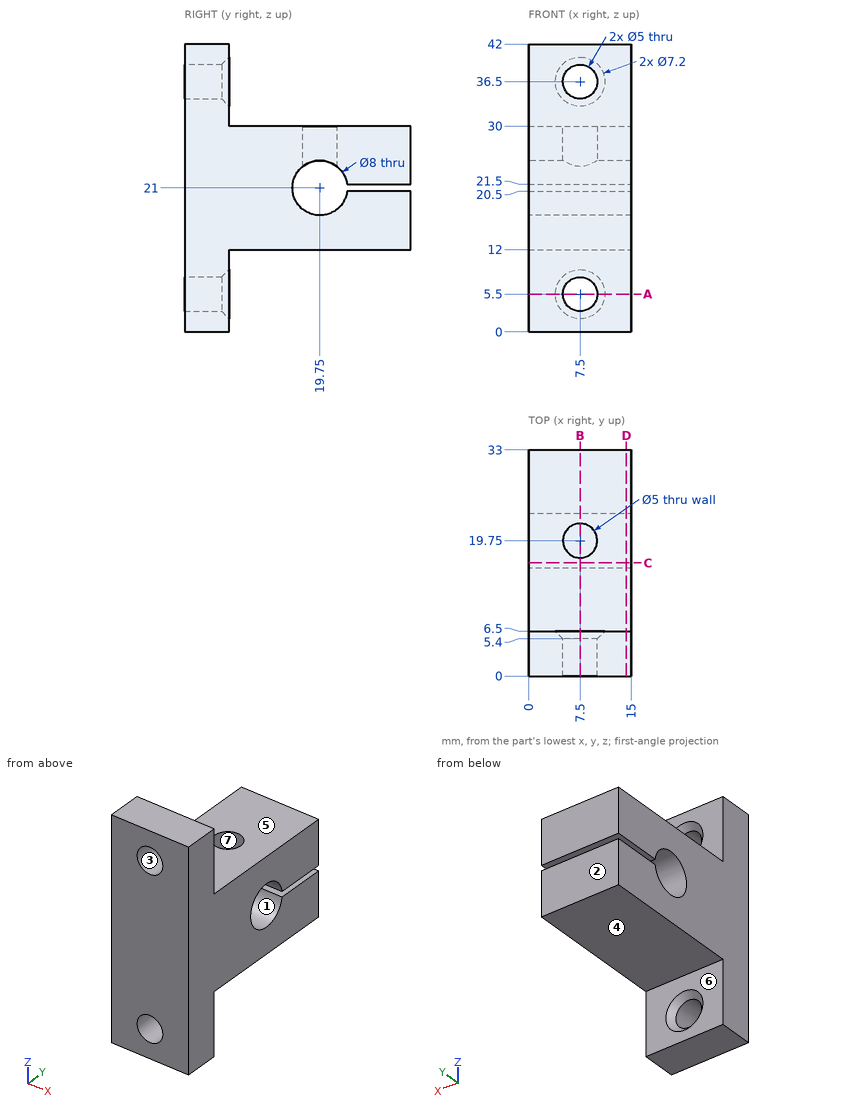
Answer from the drawing. Dimensions are ordinates in mm from the lowest x, y and z of the part. A direction names the side the tool comes from. Round coordinates to 2 decimals unless told otherwise and drop trailing zeros. Loops run counter-clockwise (first coordinate to the right, second up) from the corner with the lowest first, then second, coordinate; pieces in that order, holes last.
(1) Each of these flat-tipped pins is pushed along its axis until it touches: P1, Ø1, axis at x = 11.5, y = 28, coming from the -Z side; P2, Ø1.5, axis at x = 5.5, y = 10.5, coming from the +Z side; P3, Ø3, axis at x = 7.5, y = 19.75, coming from the +Z side. Where does it stop, or does it pass through?
Computed values:
P1: stops at z = 12
P2: stops at z = 30
P3: stops at z = 17.29
(2) The part is cut by section A-A, the plane z = 5.5. Give the vertices of the cut face in (x, y), and give its area (3 significant figures).
Computed values:
outline: (0, 0) - (5, 0) - (5, 5.4) - (3.9, 6.5) - (0, 6.5) - close; (10, 0) - (15, 0) - (15, 6.5) - (11.1, 6.5) - (10, 5.4) - close
area: 63.8 mm2
(3) The part is cut by section D-D, the plane x = 14.25. Give the vertices of the cut face in (y, z).
Computed values:
outline: (0, 0) - (6.5, 0) - (6.5, 12) - (33, 12) - (33, 20.5) - (23.72, 20.5) arc R4 cw (long way) to (23.72, 21.5) - (33, 21.5) - (33, 30) - (6.5, 30) - (6.5, 42) - (0, 42) - close
(4) Find the intervals of material crossed by L1, parallel to Z at x = 12.5, y = 25.5; L2, parallel to X at y = 2.6, z = 5.5; L3, parallel to Y at x = 5, z = 8.5, in increasing order.
Computed values:
L1: z = 12 to 20.5, 21.5 to 30
L2: x = 0 to 5, 10 to 15
L3: y = 0 to 6.5
(5) The part is cut by section B-B, the plane x = 7.5. Give the vertices of the cut face in (y, z).
Computed values:
outline: (0, 0) - (6.5, 0) - (6.5, 1.9) - (5.4, 3) - (0, 3) - close; (0, 8) - (5.4, 8) - (6.5, 9.1) - (6.5, 12) - (33, 12) - (33, 20.5) - (23.72, 20.5) arc R4 cw (long way) to (17.25, 24.12) - (17.25, 30) - (6.5, 30) - (6.5, 32.9) - (5.4, 34) - (0, 34) - close; (0, 39) - (5.4, 39) - (6.5, 40.1) - (6.5, 42) - (0, 42) - close; (22.25, 24.12) arc R4 cw to (23.72, 21.5) - (33, 21.5) - (33, 30) - (22.25, 30) - close
(6) The mould has two halves that part along Z. Classify the marked faces 1, 2, 3 and 4: pulls with the +Z half, pulls with the -Z half, needs draft (parallel to the pull), parting line crosses it, or undercut.
Computed values:
face 1: undercut
face 2: needs draft
face 3: undercut
face 4: pulls with the -Z half
(7) The part is cut by section C-C, the plane y = 16.5. Give the vertices of the cut face in (x, z).
Computed values:
outline: (0, 12) - (15, 12) - (15, 18.67) - (0, 18.67) - close; (0, 23.33) - (15, 23.33) - (15, 30) - (0, 30) - close
(8) For the marked faces 5, 6 and 7, determine the directions among +Z, -Z, +X, -X, +Y, -Y from which every point of the face is accessible in a straight line to the end or side of a thin tool.
Computed values:
face 5: +Z, +X, -X, +Y
face 6: -Z, +X, -X, +Y
face 7: +Z
